from build123d import *

# Parameters (mm, degrees)
CUT_EXTRUDE1_DEPTH = 1.3


with BuildPart() as part:
    # Sketch1 → Revolve1 (revolve)
    with BuildSketch(Plane.XY, mode=Mode.PRIVATE) as revolve1_sk:
        Polygon((0, 0), (2.75, 0), (2.75, -3), (1.5, -3), (1.5, -13), (0, -13), align=None)
    revolve(revolve1_sk.sketch.rotate(Axis((0, 0, 0), (0, -1, 0)), 180), axis=Axis((0, 0, 0), (0, -1, 0)))

    # Sketch2 → Cut-Revolve1 (revolve, cut)
    with BuildSketch(Plane.XY, mode=Mode.PRIVATE) as cut_revolve1_sk:
        Polygon((1.25, 0), (1.25, -1.3), (0, -2.021687836), (0, 0), align=None)
    revolve(cut_revolve1_sk.sketch.rotate(Axis((0, 0, 0), (0, -1, 0)), 90), axis=Axis((0, 0, 0), (0, -1, 0)), mode=Mode.SUBTRACT)

    # Sketch3 → Cut-Extrude1 (cut)
    with BuildSketch(Plane(origin=(0, 0, 0), x_dir=(1, 0, 0), z_dir=(0, 1, 0))):
        Polygon((0, 1.443375673), (-1.25, 0.721687836), (-1.25, -0.721687836), (0, -1.443375673), (1.25, -0.721687836), (1.25, 0.721687836), align=None)
    extrude(amount=-CUT_EXTRUDE1_DEPTH, mode=Mode.SUBTRACT)


solid = part.part
Read the model definition and answer for the solid it produces. Units are mm, in the model's axes. A direction names the side the tool comes from. Give positions to 0.01 mm unless a question says otherwise; leave off trailing zeros. Write each loop counter-clockwise with the first axis right and the second up, starting at its lowest first coordinate (ties: lowest second). Pieces come first, ordered by that corner, then holes. Notation, with made-up numbers: M 66.5,15.25 L 120.5,15.25 A19 cw 120.5,43.25 Z; hole C -28,-6.5 d11. An arc over 180 degrees is marked long. One line per item, written item: value. Start each with the question number.
(1) Find the intervals of material crossed by line 1 (Y direction, x = -2.1, z = 1.1); line 2 (X direction, y = -0.5, z = -1.05); line 3 (Y direction, x = -1.2, z = 0.45), in increasing order.
(2) Determine the mould class of faces 3 (the cylindrical face through (-1.43, -8.07, -0.45)), 4 (the flat face through (-1.2, -3, 1.2)), 5 (the flat face through (-0.63, -0.64, 1.08)), 6 (the flat face through (1.25, -1, 0)) for opening direction Z: pulls with the +Z half, pulls with the -Z half, needs draft (parallel to the pull), parting line crosses it, or undercut.
(3) Find section B-B (y = -4.25). Determine the outline of the cut face in (x, z), plus the area to 3 significant figures.
(4) Flat-ended cylindrical pins translate along their axes: pin 1 Ø2 at (x, y) = (1, -11.5) entering from -Z; pin 2 Ø1 at (y, z) = (-11, -1) entering from +X; pin 3 Ø1.5 at (y, z) = (-5.5, 0) entering from -X. Find the tip coordinate at first contact, or state that the pin passes through.
(5) A tool of negligible diameter and unlimited length cuts with its end or side. For faces 1 (the flat face through (0.63, -0.64, -1.08)), 2 (the cylindrical face through (0.596, -1.521, 2.685)), from which of +Z, -Z, +X, -X, +Y, -Y can it reach the whole face along a straight path? Write none if from no direction.
(6) Find section C-C (z = 2.3). Determine the outline of the cut face in (x, y).
(7) Find section D-D (x = 2.45). Determine the outline of the cut face in (y, z).
(8) Find section A-A (y = -1). Determine the outline of the cut face in (x, z).
Results below:
1. line 1: y = -3 to 0
1. line 2: x = -2.54 to -0.68, 0.68 to 2.54
1. line 3: y = -13 to -1.3
2. face 3: parting line crosses it
2. face 4: needs draft
2. face 5: undercut
2. face 6: undercut
3. outline: C 0,0 d3
3. area: 7.07 mm^2
4. pin 1: stops at z = -1.5
4. pin 2: stops at x = 1.41
4. pin 3: stops at x = -1.5
5. face 1: +Y
5. face 2: +Y, -Y
6. outline: M -1.51,-3 L 1.51,-3 L 1.51,0 L -1.51,0 Z
7. outline: M -3,-1.25 L 0,-1.25 L 0,1.25 L -3,1.25 Z
8. outline: C 0,0 d5.5; hole M -1.25,-0.72 L 0,-1.44 L 1.25,-0.72 L 1.25,0.72 L 0,1.44 L -1.25,0.72 Z
